The model under review builds one solid part; all positions refer to its coordinate system, in mm. Round coordinates to 2 decimals unless told otherwise and drop trailing zeros. Loops run counter-clockwise (first coordinate to the right, second up) from the corner with the lowest first, then second, coordinate; pieces in that order, holes last. Notation, with made-up numbers: M 82,11 L 109,11 A20 ccw 109,33 Z; hole C 69.5,5 d6. An arc over 180 degrees is marked long. Answer as a JSON object with one key per item and string values. Group by question number.
Item 1: Insertion check: P1, Ø1, axis at y = -11, z = 1.5, coming from the +X side; P2, Ø3, axis at x = 18.53, y = -31.47, coming from the -Z side. Each pin has a flat end and moves straight along its axis. Give the tip position at first contact, or say it passes through.
Item 2: Consider section B-B (x = -75). Give the boundary of the cut face in (y, z), and give its area (3 significant figures).
Item 3: Consider section D-D (y = -44.5). Give the boundary of the cut face in (x, z).
Item 4: Consider section C-C (y = 38.5). Give the boundary of the cut face in (x, z), and give its area (3 significant figures).
Item 5: To check wall thickness, follow line 1 (Y direction, x = -3.5, z = 1.95); line 2 (Y direction, x = 50, z = 0.8); line 3 (X direction, y = -20.5, z = 1.9). State the ranges of each line that lie inside material, in increasing order.
Item 6: Consider section A-A (y = 0). Give the boundary of the cut face in (x, z), and give its area (3 significant figures).
Item 7: The part is to be moulded in two halves that separate along Y. For faces 1 (the face through (-9.46, -31.03, 0.99)), 2 (the face through (1, 1, 0)), 3 (the face through (-99.988, -1.099, 0.986)), 4 (the face through (-17.66, 29.78, 1.01)), say which applies: +Y half, -Y half, draft (parallel to the pull), parting line (faces both ways), or undercut.
```python
from build123d import *

# Parameters (mm, degrees)
SKETCH_1_R          = 32.5
EXTRUDE_1_DEPTH     = 2
FILLET_1_R          = 4
SKETCH_2_R          = 1.9
CUT_EXTRUDE_1_DEPTH = 10


with BuildPart() as part:
    # 草图1 → 凸台-拉伸1 (new body)
    with BuildSketch(Plane.XY):
        with BuildLine():
            Line((-50, 50), (-25, 50))
            Line((-25, 50), (25, 50))
            Line((25, 50), (50, 50))
            ThreePointArc((50, 50), (100, 0), (50, -50))
            Line((50, -50), (25, -50))
            Line((25, -50), (-25, -50))
            Line((-25, -50), (-50, -50))
            ThreePointArc((-50, -50), (-100, 0), (-50, 50))
        make_face()
        with Locations((-50, 0)):
            Circle(SKETCH_1_R, mode=Mode.SUBTRACT)
        with Locations((50, 0)):
            Circle(SKETCH_1_R, mode=Mode.SUBTRACT)
        with BuildLine():
            Line((-6.07127469, -26.015246236), (6.07127469, -26.015246236))
            ThreePointArc((6.07127469, -26.015246236), (11.868149575, -33.948312584), (19.077305008, -40.624043109))
            Line((19.077305008, -40.624043109), (-19.077305008, -40.624043109))
            ThreePointArc((-19.077305008, -40.624043109), (-11.868149575, -33.948312584), (-6.07127469, -26.015246236))
        make_face(mode=Mode.SUBTRACT)
        with BuildLine():
            Line((19.077305008, 40.624043109), (-19.077305008, 40.624043109))
            ThreePointArc((-19.077305008, 40.624043109), (-11.868149575, 33.948312584), (-6.07127469, 26.015246236))
            Line((-6.07127469, 26.015246236), (6.07127469, 26.015246236))
            ThreePointArc((6.07127469, 26.015246236), (11.868149575, 33.948312584), (19.077305008, 40.624043109))
        make_face(mode=Mode.SUBTRACT)
    extrude(amount=EXTRUDE_1_DEPTH)

    # 圆角1
    fillet_1_edges = [part.edges().sort_by_distance(p)[0] for p in [
        (-6.07127469, -26.015246236, 1),
        (-19.077305008, -40.624043109, 1),
        (19.077305008, -40.624043109, 1),
        (6.07127469, -26.015246236, 1),
        (6.07127469, 26.015246236, 1),
        (19.077305008, 40.624043109, 1),
        (-19.077305008, 40.624043109, 1),
        (-6.07127469, 26.015246236, 1),
    ]]
    fillet(fillet_1_edges, radius=FILLET_1_R)

    # 草图2 → 切除-拉伸1 (cut)
    with BuildSketch(Plane.XY.offset(2)):
        with Locations((94.5, 0)):
            Circle(SKETCH_2_R)
        with Locations((81.466251763, -31.466251763)):
            Circle(SKETCH_2_R)
        with Locations((50, -44.5)):
            Circle(SKETCH_2_R)
        with Locations((18.533748237, -31.466251763)):
            Circle(SKETCH_2_R)
        with Locations((5.5, 0)):
            Circle(SKETCH_2_R)
        with Locations((18.533748237, 31.466251763)):
            Circle(SKETCH_2_R)
        with Locations((50, 44.5)):
            Circle(SKETCH_2_R)
        with Locations((81.466251763, 31.466251763)):
            Circle(SKETCH_2_R)
        with Locations((-81.466251763, 31.466251763)):
            Circle(SKETCH_2_R)
        with Locations((-50, 44.5)):
            Circle(SKETCH_2_R)
        with Locations((-18.533748237, 31.466251763)):
            Circle(SKETCH_2_R)
        with Locations((-5.5, 0)):
            Circle(SKETCH_2_R)
        with Locations((-18.533748237, -31.466251763)):
            Circle(SKETCH_2_R)
        with Locations((-50, -44.5)):
            Circle(SKETCH_2_R)
        with Locations((-81.466251763, -31.466251763)):
            Circle(SKETCH_2_R)
        with Locations((-94.5, 0)):
            Circle(SKETCH_2_R)
    extrude(amount=-CUT_EXTRUDE_1_DEPTH, mode=Mode.SUBTRACT)


solid = part.part
```
Geometry results:
{
 "1": {"P1": "stops at x = 98.89", "P2": "passes through"},
 "2": {"outline": "M -43.3,0 L -20.77,0 L -20.77,2 L -43.3,2 Z; M 20.77,0 L 43.3,0 L 43.3,2 L 20.77,2 Z", "area": "90.1 mm^2"},
 "3": {"outline": "M -72.8,0 L -51.9,0 L -51.9,2 L -72.8,2 Z; M -48.1,0 L 48.1,0 L 48.1,2 L -48.1,2 Z; M 51.9,0 L 72.8,0 L 72.8,2 L 51.9,2 Z"},
 "4": {"outline": "M -81.9,0 L -12.43,0 L -12.43,2 L -81.9,2 Z; M 12.43,0 L 81.9,0 L 81.9,2 L 12.43,2 Z", "area": "278 mm^2"},
 "5": {"line 1": "y = -50 to -40.62, -26.02 to 26.02, 40.62 to 50", "line 2": "y = -50 to -46.4, -42.6 to -32.5, 32.5 to 42.6, 46.4 to 50", "line 3": "x = -95.6 to -75.22, -24.78 to 24.78, 75.22 to 95.6"},
 "6": {"outline": "M -100,0 L -96.4,0 L -96.4,2 L -100,2 Z; M -92.6,0 L -82.5,0 L -82.5,2 L -92.6,2 Z; M -17.5,0 L -7.4,0 L -7.4,2 L -17.5,2 Z; M -3.6,0 L 3.6,0 L 3.6,2 L -3.6,2 Z; M 7.4,0 L 17.5,0 L 17.5,2 L 7.4,2 Z; M 82.5,0 L 92.6,0 L 92.6,2 L 82.5,2 Z; M 96.4,0 L 100,0 L 100,2 L 96.4,2 Z", "area": "110 mm^2"},
 "7": {"face 1": "undercut", "face 2": "draft", "face 3": "parting line", "face 4": "undercut"}
}
